Geometry: final body of the model. Coordinates: model frame, mm. Face numbers are marked on the shaded views. A direction names the side the tool comes from. Round coordinates to 2 decimals unless told otherwise and drop trailing zeros. Order: outer loops, then holes, each group sorted by start corner. A loop starts at its lowest first (then second) coordinate and runs counter-clockwise, first axis right, second up. Notation, with made-up numbers: (76, 56) -> (129, 56) arc R28 cw to (129, 76) -> close; hole circle Ø8 at (7.5, 44). An arc over 180 degrees is marked (long way). Put each result on its own line as item: value.
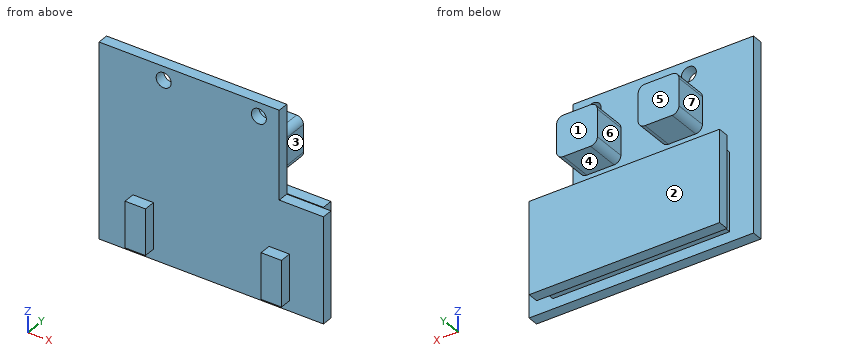
```python
from build123d import *

# Parameters (mm, degrees)
EXTRUDE_1_DEPTH     = 1.6
SKETCH_4_W          = 3
SKETCH_4_H          = 6.75
EXTRUDE_2_DEPTH     = 1.7
SKETCH_5_R          = 1.1
CUT_EXTRUDE_1_DEPTH = 22.867841686
SKETCH_6_W          = 6
SKETCH_6_H          = 6
EXTRUDE_3_DEPTH     = 5
FILLET_1_R          = 1
EXTRUDE_START       = 2
SKETCH_7_W          = 28
SKETCH_7_H          = 13.5
EXTRUDE_4_DEPTH     = 1.6
SKETCH_8_W          = 26
SKETCH_8_H          = 11.5
EXTRUDE_5_DEPTH     = 2


with BuildPart() as part:
    # Sketch 1 → Extrude 1 (new body)
    with BuildSketch(Plane(origin=(0, 0, 0), x_dir=(1, 0, 0), z_dir=(0, 1, 0))):
        Polygon((16.5, -1.25), (10, -1.25), (10, -14.25), (-16.5, -14.25), (-16.5, 14.25), (16.5, 14.25), align=None)
    extrude(amount=EXTRUDE_1_DEPTH)

    # Sketch 4 → Extrude 2 (add)
    with BuildSketch(Plane.XZ):
        with Locations((-10, -9.375)):
            Rectangle(SKETCH_4_W, SKETCH_4_H)
        with Locations((10, -9.375)):
            Rectangle(SKETCH_4_W, SKETCH_4_H)
    extrude(amount=EXTRUDE_2_DEPTH)

    # Sketch 5 → Cut-Extrude 1 (cut, through all)
    with BuildSketch(Plane(origin=(0, 0, 0), x_dir=(-1, 0, 0), z_dir=(0, -1, 0))):
        with Locations(Location((7, -12.25, 0), (0, 0, 90))):
            Circle(SKETCH_5_R)
        with Locations(Location((-7, -12.25, 0), (0, 0, 270))):
            Circle(SKETCH_5_R)
    extrude(amount=-CUT_EXTRUDE_1_DEPTH, mode=Mode.SUBTRACT)

    # Sketch 6 → Extrude 3 (add)
    with BuildSketch(Plane(origin=(0, 1.6, 0), x_dir=(1, 0, 0), z_dir=(0, 1, 0))):
        with Locations((6, -6.25)):
            Rectangle(SKETCH_6_W, SKETCH_6_H)
        with Locations((-6, -6.25)):
            Rectangle(SKETCH_6_W, SKETCH_6_H)
    extrude(amount=EXTRUDE_3_DEPTH)

    # Fillet 1
    fillet_1_edges = [part.edges().sort_by_distance(p)[0] for p in [
        (3, 4.1, 3.25),
        (3, 4.1, 9.25),
        (9, 4.1, 9.25),
        (9, 4.1, 3.25),
        (-3, 4.1, 9.25),
        (-3, 4.1, 3.25),
        (-9, 4.1, 3.25),
        (-9, 4.1, 9.25),
    ]]
    fillet(fillet_1_edges, radius=FILLET_1_R)



with BuildPart() as body_2:
    # Sketch 7 → Extrude 4 (new body)
    with BuildSketch(Plane(origin=(0, 1.6, 0), x_dir=(1, 0, 0), z_dir=(0, 1, 0)).offset(EXTRUDE_START)):
        with Locations((0, 7)):
            Rectangle(SKETCH_7_W, SKETCH_7_H)
    extrude(amount=EXTRUDE_4_DEPTH)


with BuildPart() as part_1:
    add(part.part)

    add(body_2.part)  # Extrude 5 merges body 2
    # Sketch 8 → Extrude 5 (add)
    with BuildSketch(Plane(origin=(0, 1.6, 0), x_dir=(1, 0, 0), z_dir=(0, 1, 0))):
        with Locations((0, 7)):
            Rectangle(SKETCH_8_W, SKETCH_8_H)
    extrude(amount=EXTRUDE_5_DEPTH)


solid = part_1.part
```
1. Cut plane D-D on z = -2. Return loops of the section in (x, y).
Ans:
outline: (-16.5, 0) -> (16.5, 0) -> (16.5, 1.6) -> (13, 1.6) -> (13, 3.6) -> (14, 3.6) -> (14, 5.2) -> (-14, 5.2) -> (-14, 3.6) -> (-13, 3.6) -> (-13, 1.6) -> (-16.5, 1.6) -> close
2. Cut plane A-A on z = 12.25. Return loops of the section in (x, y).
Ans:
outline: (-16.5, 0) -> (-8.1, 0) -> (-8.1, 1.6) -> (-16.5, 1.6) -> close; (-5.9, 0) -> (5.9, 0) -> (5.9, 1.6) -> (-5.9, 1.6) -> close; (8.1, 0) -> (10, 0) -> (10, 1.6) -> (8.1, 1.6) -> close
3. Material intervals for probe 1 along X at (y, z) = (0.8, 12.25); probe 2 along Z at (x, y) = (7, 0.95); probe 3 along X at (y, z) = (6, 7.25), sorted ascending.
Ans:
probe 1: -16.5 to -8.1, -5.9 to 5.9, 8.1 to 10
probe 2: -14.25 to 11.15, 13.35 to 14.25
probe 3: -9 to -3, 3 to 9
4. Cut plane C-C on x = -7. Return loops of the section in (y, z), and give its area (3 significant figures).
Ans:
outline: (0, -14.25) -> (1.6, -14.25) -> (1.6, -12.75) -> (3.6, -12.75) -> (3.6, -13.75) -> (5.2, -13.75) -> (5.2, -0.25) -> (3.6, -0.25) -> (3.6, -1.25) -> (1.6, -1.25) -> (1.6, 3.25) -> (6.6, 3.25) -> (6.6, 9.25) -> (1.6, 9.25) -> (1.6, 11.15) -> (0, 11.15) -> close; (0, 13.35) -> (1.6, 13.35) -> (1.6, 14.25) -> (0, 14.25) -> close
area: 117 mm²
5. Cut plane B-B on y = 0.5. Return loops of the section in (x, z).
Ans:
outline: (-16.5, -14.25) -> (16.5, -14.25) -> (16.5, 1.25) -> (10, 1.25) -> (10, 14.25) -> (-16.5, 14.25) -> close; hole circle Ø2.2 at (-7, 12.25); hole circle Ø2.2 at (7, 12.25)
6. Draft query along X for the marked faces 5, 6 and 7. Return one class per face: +X half, -X half, draft (parallel to the pull), parting line (faces both ways), or undercut.
Ans:
face 5: draft
face 6: undercut
face 7: -X half
7. Set-up query: the marked faces 1, 2, 3 and 4. Return all of +Z, -Z, +X, -X, +Y, -Y with unobstructed straight access to the full face (end or side cutting, diameter ignored); none if empty.
Ans:
face 1: +Z, -Z, +X, -X, +Y
face 2: -Z, +X, -X, +Y
face 3: +Z, +X, +Y
face 4: +X, -X, +Y
8. Contact query for flat-ended pins moving along their axis: P1, Ø1, axis at x = 4, y = 4, coming from the -Z side; P2, Ø3, axis at y = 4.5, z = 7, coming from the -X side; P3, Ø1.8, axis at y = 0.5, z = 10.5, coming from the +X side. Output: stop coordinate, or through.
Ans:
P1: z = -13.75
P2: x = -9
P3: x = 10
